```python
from build123d import *

# Parameters (mm, degrees)
SALIENTE_EXTRUIR1_DEPTH = 8
CROQUIS6_W              = 152
CROQUIS6_H              = 1.5
CORTAR_EXTRUIR10_DEPTH  = 1.5
CORTAR_EXTRUIR12_DEPTH  = 128
CROQUIS12_W             = 24
CROQUIS12_H             = 5.5
CORTAR_EXTRUIR13_DEPTH  = 1.5
CORTAR_EXTRUIR14_DEPTH  = 5.5
CORTAR_EXTRUIR16_DEPTH  = 1.5
CROQUIS17_W             = 76
CROQUIS17_H             = 4
CORTAR_EXTRUIR17_DEPTH  = 18
CROQUIS18_W             = 10
CROQUIS18_H             = 5.5
CORTAR_EXTRUIR18_DEPTH  = 1
CORTAR_EXTRUIR22_DEPTH  = 5
CORTAR_EXTRUIR23_DEPTH  = 0.5
CORTAR_EXTRUIR25_DEPTH  = 1.5
SALIENTE_EXTRUIR3_DEPTH = 1.5
SALIENTE_EXTRUIR4_DEPTH = 1.5


with BuildPart() as part:
    # Croquis2 → Saliente-Extruir1 (new body)
    with BuildSketch(Plane.XY):
        Polygon((0, 0), (240, 0), (240, 48), (228, 48), (228, 65), (152, 65), (152, 50), (0, 50), align=None)
    extrude(amount=SALIENTE_EXTRUIR1_DEPTH)

    # Croquis6 → Cortar-Extruir10 (cut)
    with BuildSketch(Plane(origin=(0, 50, 0), x_dir=(1, 0, 0), z_dir=(0, 1, 0))):
        with Locations((76, -6.25)):
            Rectangle(CROQUIS6_W, CROQUIS6_H)
    extrude(amount=-CORTAR_EXTRUIR10_DEPTH, mode=Mode.SUBTRACT)

    # Croquis9 → Cortar-Extruir12 (cut)
    with BuildSketch(Plane.ZY):
        Polygon((5.5, 48.5), (5.5, 46.5), (6.5, 46.5), (6.5, 45), (0, 45), (0, 50), (5.5, 50), align=None)
    extrude(amount=-CORTAR_EXTRUIR12_DEPTH, mode=Mode.SUBTRACT)

    # Croquis12 → Cortar-Extruir13 (cut)
    with BuildSketch(Plane(origin=(0, 50, 0), x_dir=(1, 0, 0), z_dir=(0, 1, 0))):
        with Locations((140, -2.75)):
            Rectangle(CROQUIS12_W, CROQUIS12_H)
    extrude(amount=-CORTAR_EXTRUIR13_DEPTH, mode=Mode.SUBTRACT)

    # Croquis13 → Cortar-Extruir14 (cut)
    with BuildSketch(Plane(origin=(0, 0, 0), x_dir=(-1, 0, 0), z_dir=(0, 0, -1))):
        Polygon((-142, 48.5), (-128, 45), (-128, 48.5), align=None)
    extrude(amount=-CORTAR_EXTRUIR14_DEPTH, mode=Mode.SUBTRACT)

    # Croquis14 → Cortar-Extruir16 (cut)
    with BuildSketch(Plane(origin=(0, 0, 5.5), x_dir=(-1, 0, 0), z_dir=(0, 0, -1))):
        Polygon((-128, 45), (-128, 46.5), (-134, 46.5), align=None)
    extrude(amount=-CORTAR_EXTRUIR16_DEPTH, mode=Mode.SUBTRACT)

    # Croquis17 → Cortar-Extruir17 (cut)
    with BuildSketch(Plane(origin=(0, 65, 0), x_dir=(1, 0, 0), z_dir=(0, 1, 0))):
        with Locations((190, -2)):
            Rectangle(CROQUIS17_W, CROQUIS17_H)
    extrude(amount=-CORTAR_EXTRUIR17_DEPTH, mode=Mode.SUBTRACT)

    # Croquis18 → Cortar-Extruir18 (cut)
    with BuildSketch(Plane(origin=(0, 48.5, 0), x_dir=(1, 0, 0), z_dir=(0, 1, 0))):
        with Locations((147, -2.75)):
            Rectangle(CROQUIS18_W, CROQUIS18_H)
    extrude(amount=-CORTAR_EXTRUIR18_DEPTH, mode=Mode.SUBTRACT)

    # Croquis19 → Cortar-Extruir22 (cut)
    with BuildSketch(Plane(origin=(0, 0, 0), x_dir=(-1, 0, 0), z_dir=(0, 0, -1))):
        Polygon((-142, 47.5), (-128, 45), (-142, 48.5), align=None)
    extrude(amount=-CORTAR_EXTRUIR22_DEPTH, mode=Mode.SUBTRACT)

    # Croquis20 → Cortar-Extruir23 (cut)
    with BuildSketch(Plane(origin=(0, 0, 5), x_dir=(-1, 0, 0), z_dir=(0, 0, -1))):
        Polygon((-142, 48.5), (-142, 47.5), (-128, 45), align=None)
    extrude(amount=-CORTAR_EXTRUIR23_DEPTH, mode=Mode.SUBTRACT)

    # Croquis21 → Cortar-Extruir25 (cut)
    with BuildSketch(Plane(origin=(0, 0, 5.5), x_dir=(-1, 0, 0), z_dir=(0, 0, -1))):
        Polygon((-134, 46.5), (-136.4, 46.5), (-134, 46.071428571), (-128, 45), align=None)
    extrude(amount=-CORTAR_EXTRUIR25_DEPTH, mode=Mode.SUBTRACT)

    # Croquis22 → Saliente-Extruir3 (add)
    with BuildSketch(Plane(origin=(240, 0, 0), x_dir=(0, 0, -1), z_dir=(1, 0, 0))):
        Polygon((0, 48), (0, 54), (-7, 48), align=None)
    extrude(amount=-SALIENTE_EXTRUIR3_DEPTH)

    # Croquis23 → Saliente-Extruir4 (add)
    with BuildSketch(Plane.ZY):
        Polygon((0, 50), (0, 56), (7, 50), (7, 48.5), (5.5, 48.5), (5.5, 46.5), (6.5, 46.5), (6.5, 45), (0, 45), align=None)
    extrude(amount=-SALIENTE_EXTRUIR4_DEPTH)


solid = part.part
```
Geometry check sheet. Reference: the model listing, model coordinates, mm. A direction names the side the tool comes from. Coordinates: 2 decimals unless noted, no trailing zeros. Write each loop counter-clockwise with the first axis right and the second up, starting at its lowest first coordinate (ties: lowest second). Pieces come first, ordered by that corner, then holes. Notation, with made-up numbers: M -22,-37 L 37,-37 A22 cw 37,-9 Z; hole C -17,51 d5. An arc over 180 degrees is marked long. One line per item, written item: value. Start each with the question number.
(1) Scan lines: line 1 along X through (y, z) = (52.5, 1); line 2 along Y through (x, z) = (64.5, 3); line 3 along Y through (x, z) = (208, 3.25). Record each from-to range of solid material in increasing order. Write a range as [from, to].
(2) Sectioned sample at C-C, the plane x = 200. Enter the section's corners in (y, z).
(3) Sectioned sample at A-A, the plane x = 102.5. Enter the section's corners in (y, z), and give its area (3 significant figures).
(4) Release check for a two-part mould opening along X. For faces 1 (the face through (240, 27, 4)), 2 (the face through (189, 47, 2)), 3 (the face through (239.3, 51, 3.5)), 4 (the face through (0, 28, 4)) record: released by +X, released by -X, zero draft, split by the parting line, or undercut.
(5) Sectioned sample at B-B, the plane z = 1.75. Enter the section's corners in (x, y), and give its area (3 significant figures).
(6) Depth check by flat-ended pin: pin 1 (1.2 mm diameter, centred on y = 53, z = 6.5, fed in from -X); pin 2 (4 mm diameter, centred on x = 235.5, z = 5, fed in from +Y); pin 3 (4.5 mm diameter, centred on y = 55.5, z = 7, fed in from +X). Enter the tip coordinate at first touch or a pass-through.
(7) Tool access check on faces 5 (the face through (0.7, 53, 3.5)), 6 (the face through (238.5, 50, 2)), 7 (the face through (147, 47.5, 3)). Record the directions out of +Z, -Z, +X, -X, +Y, -Y that give a thin tool (end or side, any length) a straight path to the whole face; none if there is none.
Filled sheet:
1. line 1: [0, 1.5], [238.5, 240]
1. line 2: [0, 45]
1. line 3: [0, 47]
2. outline: M 0,0 L 47,0 L 47,4 L 65,4 L 65,8 L 0,8 Z
3. outline: M 0,0 L 45,0 L 45,6.5 L 46.5,6.5 L 46.5,5.5 L 48.5,5.5 L 48.5,7 L 50,7 L 50,8 L 0,8 Z
3. area: 369 mm²
4. face 1: released by +X
4. face 2: undercut
4. face 3: zero draft
4. face 4: released by -X
5. outline: M 0,0 L 240,0 L 240,52.5 L 238.5,52.5 L 238.5,48 L 228,48 L 228,47 L 152,47 L 152,47.5 L 142,47.5 L 128,45 L 1.5,45 L 1.5,54.5 L 0,54.5 Z
5. area: 11,100 mm²
6. pin 1: x = 152
6. pin 2: y = 48
6. pin 3: x = 228
7. face 5: +Z, -X, +Y
7. face 6: +Z, -Z, +Y
7. face 7: -Z, +Y
